Source: CAD feature listing. Evaluate the final solid. Frame: model axes, mm. Coordinates: 2 decimals unless noted, no trailing zeros. Order: outer loops, then holes, each group sorted by start corner. A loop starts at its lowest first (then second) coordinate and runs counter-clockwise, first axis right, second up.
Item 1: Mould query, pull axis X, two halves, no side actions, for faces 1 (the cylindrical face through (-9.873, -25.324, 0.507)), 2 (the cylindrical face through (9.9, -25.303, 0.507)), 3 (the flat face through (-16.1, -18.1, 1)). Classes: released by +X, released by -X, zero draft, split by the parting line, or undercut.
Item 2: Section C-C on x = 18. Return the cut outline in (y, z), then the cut area to 3 significant figures.
Item 3: Section A-A on y = 7.5. Return the cut outline in (x, z).
Item 4: Ray query, line 1 (X direction, y = 0, z = 0.6); line 2 (Y direction, x = 8, z = 0.2); line 3 (X direction, y = 4, z = 0.15). Return the intervals inside material, ascending.
Item 5: Section B-B on z = 0.35. Return the cut outline in (x, y).
Item 6: Section D-D on x = 0. Return the cut outline in (y, z), then the cut area to 3 significant figures.
from build123d import *

# Parameters (mm, degrees)
F1_DEPTH = 1
F2_R     = 1
F3_R     = 1
F4_D     = 1
F4_DEPTH = 2
F4_TIP   = 0.3004303095
F5_R     = 5
F6_R     = 5


with BuildPart() as f1:
    # F0 (on Top) → F1 (new body)
    with BuildSketch(Plane.XY):
        with BuildLine():
            Line((-2.5, -34.5), (-2.5, -26.8840101175))
            ThreePointArc((-2.5, -26.8840101175), (-6.224328148, -26.2727565951), (-9.8270364159, -25.1481481481))
            Line((-9.8270364159, -25.1481481481), (-6.1635182079, -29.8240740741))
            Line((-6.1635182079, -29.8240740741), (-2.5, -34.5))
        make_face()
        with BuildLine():
            ThreePointArc((9.8270364159, -25.1481481481), (6.224328148, -26.2727565951), (2.5, -26.8840101175))
            Line((2.5, -26.8840101175), (2.5, -34.5))
            Line((2.5, -34.5), (6.1635182079, -29.8240740741))
            Line((6.1635182079, -29.8240740741), (9.8270364159, -25.1481481481))
        make_face()
        with BuildLine():
            Line((-2.5, -26.8840101175), (-2.5, -26.5288885241))
            Line((-2.5, -26.5288885241), (-9.8270364159, -25.1481481481))
            ThreePointArc((-9.8270364159, -25.1481481481), (-6.224328148, -26.2727565951), (-2.5, -26.8840101175))
        make_face()
        with BuildLine():
            Line((9.8270364159, -25.1481481481), (2.5, -26.5288885241))
            Line((2.5, -26.5288885241), (2.5, -26.8840101175))
            ThreePointArc((2.5, -26.8840101175), (6.224328148, -26.2727565951), (9.8270364159, -25.1481481481))
        make_face()
        with BuildLine():
            ThreePointArc((-2.5, -23.8694365246), (-16.0623784042, 17.8325545001), (24, 0))
            ThreePointArc((24, 0), (17.8325545001, -16.0623784042), (2.5, -23.8694365246))
            Line((2.5, -23.8694365246), (2.5, -26.5288885241))
            Line((2.5, -26.5288885241), (9.8270364159, -25.1481481481))
            ThreePointArc((9.8270364159, -25.1481481481), (22.2971969452, -15.2261291334), (27, 0))
            ThreePointArc((27, 0), (-15.2261291334, 22.2971969452), (-9.8270364159, -25.1481481481))
            Line((-9.8270364159, -25.1481481481), (-2.5, -26.5288885241))
            Line((-2.5, -26.5288885241), (-2.5, -23.8694365246))
        make_face()
    extrude(amount=F1_DEPTH)

    # F2
    f2_edges = [f1.edges().sort_by_distance(p)[0] for p in [
        (2.5, -34.5, 0.5),
    ]]
    fillet(f2_edges, radius=F2_R)

    # F3
    f3_edges = [f1.edges().sort_by_distance(p)[0] for p in [
        (-2.5, -34.5, 0.5),
    ]]
    fillet(f3_edges, radius=F3_R)

    # F4
    with Locations(Plane(origin=(0, 0, 0), x_dir=(1, 0, 0), z_dir=(0, 0, -1))):
        with Locations((-4.5891780847, 28.5906020734), (4.5891780847, 28.5906020734)):
            Hole(F4_D / 2, depth=F4_DEPTH)
            with Locations((0, 0, -(F4_DEPTH + F4_TIP / 2))):  # 118° drill point
                Cone(0, F4_D / 2, F4_TIP, mode=Mode.SUBTRACT)

    # F5
    f5_edges = [f1.edges().sort_by_distance(p)[0] for p in [
        (-9.827036, -25.148148, 0.5),
    ]]
    fillet(f5_edges, radius=F5_R)

    # F6
    f6_edges = [f1.edges().sort_by_distance(p)[0] for p in [
        (9.827036, -25.148148, 0.5),
    ]]
    fillet(f6_edges, radius=F6_R)


solid = f1.part
Answer list:
1. face 1: released by -X
1. face 2: released by +X
1. face 3: zero draft
2. outline: (-20.12, 0) - (-15.87, 0) - (-15.87, 1) - (-20.12, 1) - close; (15.87, 0) - (20.12, 0) - (20.12, 1) - (15.87, 1) - close
2. area: 8.50 mm2
3. outline: (-25.94, 0) - (-22.8, 0) - (-22.8, 1) - (-25.94, 1) - close; (22.8, 0) - (25.94, 0) - (25.94, 1) - (22.8, 1) - close
4. line 1: x = -27 to -24, 24 to 27
4. line 2: y = -27.48 to -22.63, 22.63 to 25.79
4. line 3: x = -26.7 to -23.66, 23.66 to 26.7
5. outline: (-10.93, -24.69) arc R5 cw to (-9.02, -26.18) - (-4.29, -32.22) arc R1 ccw to (-2.5, -31.6) - (-2.5, -23.87) arc R24 cw (long way) to (2.5, -23.87) - (2.5, -31.6) arc R1 ccw to (4.29, -32.22) - (9.02, -26.18) arc R5 cw to (10.93, -24.69) arc R27 ccw (long way) to start; hole circle Ø1 at (-4.59, -28.59); hole circle Ø1 at (4.59, -28.59)
6. outline: (24, 0) - (27, 0) - (27, 1) - (24, 1) - close
6. area: 3.00 mm2
